For this review, take the finished solid that the model builds, in its own axes (mm). Give positions to 0.01 mm unless a question says otherwise; leave off trailing zeros. Write each loop counter-clockwise with the first axis right and the second up, starting at its lowest first coordinate (ties: lowest second). Pieces come first, ordered by that corner, then holes. Notation, with made-up numbers: M -26,69.25 L 6,69.25 A25 ccw 6,87.25 Z; hole C 78,-27.5 d9. An arc over 180 degrees is marked long. One line per item, written item: value. Start each with the question number.
Item 1: Clearance check with a flat-ended pin moving along its axis: pin 1 Ø23 at (x, y) = (0, 25.4) entering from +Z (3 decimals). State where the tip first meets the part, or that it passes through.
Item 2: Consider section D-D, the plane y = -33. Write out the cut boundary in (x, z) (3 decimals), and give its area (3 significant figures).
Item 3: Consider section C-C, the plane z = -1.1. Write out the cut boundary in (x, y).
Item 4: Consider section A-A, the plane x = 0. Write out the cut boundary in (y, z) (3 decimals).
Item 5: Consider section B-B, the plane y = 25.4. Write out the cut boundary in (x, z) (3 decimals).
Item 6: To check wall thickness, follow probe 1 along Y at (x, z) = (0, -1.6); probe 2 along Y at (x, z) = (3.5, -0.65); probe 3 along X at (y, z) = (-51.5, -0.4). State the ranges of each line that lie inside material, in increasing order.
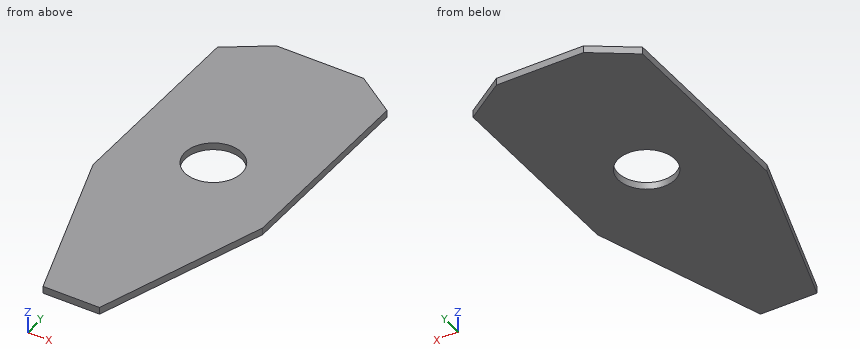
```python
from build123d import *

# Parameters (mm, degrees)
F0_R     = 12.7
F1_DEPTH = 3.175


# Not quite as in the source:
# - a length typed as a fraction of an inch, garbled in the dataset ("3 / 203.2 mm" for 3/8 in), is restored


with BuildPart() as f1:
    # F0 (on Top) → F1 (new body)
    with BuildSketch(Plane.XY):
        Polygon((-38.1, 0), (-12.7, -76.2), (12.7, -76.2), (38.1, 0), (38.1, 50.8), (38.1, 88.9), (19.6133758873, 101.6), (-19.6133758873, 101.6), (-38.1, 88.9), (-38.1, 50.8), align=None)
        with Locations((0, 25.4)):
            Circle(F0_R, mode=Mode.SUBTRACT)
    extrude(amount=-F1_DEPTH)


solid = f1.part
```
Model answer:
1. pin 1: passes through
2. outline: M -27.1,-3.175 L 27.1,-3.175 L 27.1,0 L -27.1,0 Z
2. area: 172 mm2
3. outline: M -38.1,0 L -12.7,-76.2 L 12.7,-76.2 L 38.1,0 L 38.1,88.9 L 19.61,101.6 L -19.61,101.6 L -38.1,88.9 Z; hole C 0,25.4 d25.4
4. outline: M -76.2,-3.175 L 12.7,-3.175 L 12.7,0 L -76.2,0 Z; M 38.1,-3.175 L 101.6,-3.175 L 101.6,0 L 38.1,0 Z
5. outline: M -38.1,-3.175 L -12.7,-3.175 L -12.7,0 L -38.1,0 Z; M 12.7,-3.175 L 38.1,-3.175 L 38.1,0 L 12.7,0 Z
6. probe 1: y = -76.2 to 12.7, 38.1 to 101.6
6. probe 2: y = -76.2 to 13.19, 37.61 to 101.6
6. probe 3: x = -20.93 to 20.93
